from build123d import *

# Parameters (mm, degrees)
BOSS_EXTRU_5_DEPTH       = 50
ESQUISSE5_R              = 2.15
ESQUISSE5_W              = 23.2
ESQUISSE5_H              = 31.8
ENL_V_MAT_EXTRU_1_DEPTH  = 10
BOSS_EXTRU_6_DEPTH       = 5
ESQUISSE9_W              = 102
ESQUISSE9_H              = 34.999999956
ENL_V_MAT_EXTRU_2_DEPTH  = 81
ESQUISSE11_R             = 2.5
ENL_V_MAT_EXTRU_9_DEPTH  = 5
ENL_V_MAT_EXTRU_12_DEPTH = 12
CONG_1_R                 = 10
ESQUISSE12_W             = 31
ESQUISSE12_H             = 23.2
ENL_V_MAT_EXTRU_13_DEPTH = 10
CONG_2_R                 = 1


with BuildPart() as part:
    # Esquisse1 → Boss.-Extru.5 (new body, symmetric)
    with BuildSketch(Plane(origin=(0, 0, 0), x_dir=(1, 0, 0), z_dir=(0, 1, 0))):
        with BuildLine():
            ThreePointArc((-36.124783736, -31), (-19.557607216, -42.100955404), (0, -46))
            Line((0, -46), (0, -51))
            ThreePointArc((0, -51), (-19.557607216, -47.100955404), (-36.124783736, -36))
            Line((-36.124783736, -36), (-80, -36))
            Line((-80, -36), (-80, 36))
            Line((-80, 36), (-36.124783736, 36))
            ThreePointArc((-36.124783736, 36), (-19.557607216, 47.100955404), (0, 51))
            Line((0, 51), (0, 46))
            ThreePointArc((0, 46), (-19.557607216, 42.100955404), (-36.124783736, 31))
            Line((-36.124783736, 31), (-70, 31))
            Line((-70, 31), (-70, -31))
            Line((-70, -31), (-36.124783736, -31))
        make_face()
    extrude(amount=BOSS_EXTRU_5_DEPTH, both=True)

    # Esquisse5 → Enlèv. mat.-Extru.1 (cut)
    with BuildSketch(Plane(origin=(-70, 0, 0), x_dir=(0, 0, -1), z_dir=(1, 0, 0))):
        with BuildLine():
            Line((-11.59999996, -2), (11.60000004, -2))
            Line((11.60000004, -2), (11.60000004, 5.500000044))
            ThreePointArc((11.60000004, 5.500000044), (10.281980555, 8.68198056), (7.10000004, 10.000000044))
            Line((7.10000004, 10.000000044), (-7.099999871, 10.000000044))
            ThreePointArc((-7.099999871, 10.000000044), (-10.281980449, 8.681980534), (-11.59999996, 5.499999956))
            Line((-11.59999996, 5.499999956), (-11.59999996, -2))
        make_face()
        Circle(ESQUISSE5_R, mode=Mode.SUBTRACT)
        Circle(ESQUISSE5_R)
        with Locations((4e-08, -17.9)):
            Rectangle(ESQUISSE5_W, ESQUISSE5_H)
        with BuildLine():
            ThreePointArc((2.15, 0), (-1.209582286, 1.77747312), (-0.788986692, -2))
            Line((-0.788986692, -2), (0.788986692, -2))
            ThreePointArc((0.788986692, -2), (1.77747312, -1.209582286), (2.15, 0))
        make_face()
        with BuildLine():
            Line((0.788986692, -2), (-0.788986692, -2))
            ThreePointArc((-0.788986692, -2), (0, -2.15), (0.788986692, -2))
        make_face()
    extrude(amount=-ENL_V_MAT_EXTRU_1_DEPTH, mode=Mode.SUBTRACT)

    # Esquisse8 → Boss.-Extru.6 (add)
    with BuildSketch(Plane(origin=(0, -50, 0), x_dir=(1, 0, 0), z_dir=(0, 1, 0))):
        with BuildLine():
            Line((0, -51), (0, 51))
            ThreePointArc((0, 51), (-19.557607216, 47.100955404), (-36.124783736, 36))
            Line((-36.124783736, 36), (-80, 36))
            Line((-80, 36), (-80, -36))
            Line((-80, -36), (-36.124783736, -36))
            ThreePointArc((-36.124783736, -36), (-19.557607216, -47.100955404), (0, -51))
        make_face()
    extrude(amount=-BOSS_EXTRU_6_DEPTH)

    # Esquisse9 → Enlèv. mat.-Extru.2 (cut, through all)
    with BuildSketch(Plane(origin=(0, 0, 0), x_dir=(0, 0, -1), z_dir=(1, 0, 0))):
        with Locations((0, 32.500000022)):
            Rectangle(ESQUISSE9_W, ESQUISSE9_H)
    extrude(amount=-ENL_V_MAT_EXTRU_2_DEPTH, mode=Mode.SUBTRACT)

    # Esquisse11 → Enlèv. mat.-Extru.9 (cut)
    with BuildSketch(Plane(origin=(-70, 0, 0), x_dir=(0, 0, -1), z_dir=(1, 0, 0))):
        with Locations((-19.59999996, -22.213953621)):
            Circle(ESQUISSE11_R)
        with Locations((19.59999996, -22.213953621)):
            Circle(ESQUISSE11_R)
    extrude(amount=-ENL_V_MAT_EXTRU_9_DEPTH, mode=Mode.SUBTRACT)

    # Esquisse10 → Enlèv. mat.-Extru.12 (cut)
    with BuildSketch(Plane(origin=(0, 0, 0), x_dir=(0, 0, -1), z_dir=(1, 0, 0))):
        with BuildLine():
            Line((136.28713183, 33.486696785), (85.263165158, 65.69401727))
            ThreePointArc((85.263165158, 65.69401727), (69.088826466, 48.564130721), (49.552191154, 35.397425514))
            ThreePointArc((49.552191154, 35.397425514), (-14.729470129, 24.226140009), (-73.513371624, 52.534840476))
            ThreePointArc((-73.513371624, 52.534840476), (-79.660455319, 58.871393898), (-85.263165158, 65.69401727))
            Line((-85.263165158, 65.69401727), (-136.28713183, 33.486696785))
            ThreePointArc((-136.28713183, 33.486696785), (-98.721588704, -4.696131807), (-51, -29.022011055))
            Line((-51, -29.022011055), (-51, 15.000000044))
            Line((-51, 15.000000044), (-46, 15.000000044))
            Line((-46, 15.000000044), (-46, -30.539714713))
            ThreePointArc((-46, -30.539714713), (0, -37), (46, -30.539714713))
            Line((46, -30.539714713), (46, 15.000000044))
            Line((46, 15.000000044), (51, 15.000000044))
            Line((51, 15.000000044), (51, -29.022011055))
            ThreePointArc((51, -29.022011055), (98.721588704, -4.696131807), (136.28713183, 33.486696785))
        make_face()
        with BuildLine():
            ThreePointArc((-51, -29.022011055), (-48.505936298, -29.800419724), (-46, -30.539714713))
            Line((-46, -30.539714713), (-46, 15.000000044))
            Line((-46, 15.000000044), (-51, 15.000000044))
            Line((-51, 15.000000044), (-51, -29.022011055))
        make_face()
        with BuildLine():
            ThreePointArc((46, -30.539714713), (48.505936298, -29.800419724), (51, -29.022011055))
            Line((51, -29.022011055), (51, 15.000000044))
            Line((51, 15.000000044), (46, 15.000000044))
            Line((46, 15.000000044), (46, -30.539714713))
        make_face()
    extrude(amount=-ENL_V_MAT_EXTRU_12_DEPTH, mode=Mode.SUBTRACT)

    # Congé1
    cong_1_edges = [part.edges().sort_by_distance(p)[0] for p in [
        (-80, -19.999999978, 36),
        (-80, -19.999999978, -36),
    ]]
    fillet(cong_1_edges, radius=CONG_1_R)

    # Esquisse12 → Enlèv. mat.-Extru.13 (cut)
    with BuildSketch(Plane(origin=(0, -55, 0), x_dir=(-1, 0, 0), z_dir=(0, -1, 0))):
        with Locations((15.5, 0)):
            Rectangle(ESQUISSE12_W, ESQUISSE12_H)
    extrude(amount=-ENL_V_MAT_EXTRU_13_DEPTH, mode=Mode.SUBTRACT)

    # Congé2
    cong_2_edges = [part.edges().sort_by_distance(p)[0] for p in [
        (-15.5, -50, -11.6),
        (-31, -50, 0),
        (-15.5, -50, 11.6),
    ]]
    fillet(cong_2_edges, radius=CONG_2_R)


solid = part.part
Part model, mm, in its own coordinate system. A direction names the side the tool comes from. Coordinates: 2 decimals unless noted, no trailing zeros. Order: outer loops, then holes, each group sorted by start corner. A loop starts at its lowest first (then second) coordinate and runs counter-clockwise, first axis right, second up. Notation, with made-up numbers: (8.5, 6.5) - (16.5, 6.5) arc R19 cw to (16.5, 11.5) - close; hole circle Ø2 at (12.5, 77). An arc over 180 degrees is marked (long way). Use CSV: the item, a comma, the result in double quotes.
Item 1: Probe probe 1 along Z at (x, y) = (-56.5, -4); probe 2 along Y at (x, z) = (-73.75, 19.6); probe 3 along Y at (x, z) = (-66.5, 3). List the from-to ranges inside material, lowest first.
Solved:
probe 1,"z = -36 to -31, 31 to 36"
probe 2,"y = -55 to -24.71, -19.71 to 15"
probe 3,"y = -55 to -50"
Item 2: Saw through at C-C on z = 2. Give the cut face in (x, y), and give its area (3 significant figures).
Solved:
outline,"(-80, -55) - (-31, -55) - (-31, -51) arc R1 ccw to (-32, -50) - (-70, -50) - (-70, -33.8) - (-80, -33.8) - close; (-80, 10) - (-70, 10) - (-70, 15) - (-80, 15) - close"
area,"457 mm²"
Item 3: Saw through at B-B on x = -24. Give the cut face in (y, z), and give its area (3 significant figures).
Solved:
outline,"(-55, -45) - (15, -45) - (15, -40) - (-50, -40) - (-50, -12.6) arc R1 ccw to (-51, -11.6) - (-55, -11.6) - close; (-55, 11.6) - (-51, 11.6) arc R1 ccw to (-50, 12.6) - (-50, 40) - (15, 40) - (15, 45) - (-55, 45) - close"
area,"984 mm²"
Item 4: Drop flat-ended pins along their axis: P1, Ø4, axis at y = -22, z = 19, coming from the +X side; P2, Ø4, axis at y = -18, z = -29.5, coming from the -X side; P3, Ø5, axis at x = -30.5, z = 22.5, coming from the +Y side. Give the stop position or say it passes through.
Solved:
P1,"stops at x = -70"
P2,"stops at x = -79.89"
P3,"stops at y = -50"
Item 5: 3-axis set-ups, long thin cutter, end or side, ignore diameter. For faces 1 (the face through (-75, -22, -20)), 2 (the face through (-53, -17, -31)), 3 (the face through (-53, -20, -36)): which of +Z, -Z, +X, -X, +Y, -Y reach the whole face in a straight line?
Solved:
face 1,"+X"
face 2,"+X, +Y"
face 3,"-Z, -X, +Y, -Y"
Item 6: Saw through at D-D on y = -48.5. Give the cut face in (x, z), and give its area (3 significant figures).
Solved:
outline,"(-80, -26) arc R10 ccw to (-70, -36) - (-36.12, -36) arc R51 ccw to (0, -51) - (0, -46) arc R51 cw to (-36.12, -31) - (-70, -31) - (-70, 31) - (-36.12, 31) arc R51 cw to (0, 46) - (0, 51) arc R51 ccw to (-36.12, 36) - (-70, 36) arc R10 ccw to (-80, 26) - close"
area,"1,380 mm²"
Item 7: Mould opens along Y. For faces 4 (the face through (-72.46, -23.17, -21.91)), 5 (the face through (-41, -55, -1)), 6 (the face through (-53, -17, 31)) say: +Y half, -Y half, draft (parallel to the pull), parting line (faces both ways), or undercut.
Solved:
face 4,"undercut"
face 5,"-Y half"
face 6,"draft"
Item 8: Saw through at A-A on y = -2. Give the cut face in (x, z), and give its area (3 significant figures).
Solved:
outline,"(-80, -26) arc R10 ccw to (-70, -36) - (-36.12, -36) arc R51 ccw to (-12, -49.57) - (-12, -44.57) arc R51 cw to (-36.12, -31) - (-70, -31) - (-70, -11.6) - (-80, -11.6) - close; (-80, 11.6) - (-70, 11.6) - (-70, 31) - (-36.12, 31) arc R51 cw to (-12, 44.57) - (-12, 49.57) arc R51 ccw to (-36.12, 36) - (-70, 36) arc R10 ccw to (-80, 26) - close"
area,"1,030 mm²"
